Here's how the part is built. I have some questions about the finished solid (model axes, mm). Face numbers are marked on the shaded views. Round coordinates to 2 decimals unless told otherwise and drop trailing zeros. Write each loop counter-clockwise with the first axis right and the second up, starting at its lowest first coordinate (ties: lowest second). Pieces come first, ordered by that corner, then holes. Notation, with made-up numbers: M -12.5,32.5 L 15.5,32.5 A19 cw 15.5,54.5 Z; hole C -10,72.5 d1. An arc over 180 degrees is marked long. Use one line per item in the form item = value. Start each with the question number.
Q1. I want a section at A-A on z = 0. List the corners of the cut face in (x, y) for me.
Q2. I'm going to push flat-ended pins straight in: pin 1 Ø10 at (x, y) = (16.5, 10) entering from +Z; pin 2 Ø6 at (x, y) = (-25, 31) entering from +Z; pin 3 Ø6 at (x, z) = (0, 0) entering from -Y. Where does each tip first touch, or does it pass through?
Q3. I want a section at C-C on x = 16. List the corners of the cut face in (y, z) for me, and give its area (3 significant figures).
Q4. I want a section at D-D on y = 32.5. List the corners of the cut face in (x, z) for me, and give its area (3 significant figures).
Q5. I need wall thicknesses on line 1 along X through (y, z) = (37.25, 0); line 2 along X through (y, z) = (7, 0); line 3 along X through (y, z) = (23, 1). Which ranges of each line are inside material? Lowest first, please. Write a range as from..to.
Q6. We'd pull the mould along Z, two halves only. Please class the marked faces 1, 2, 3 and 4: +Z half, -Z half, draft (parallel to the pull), parting line (faces both ways), or undercut.
Q7. I want a section at B-B on y = 47. List the corners of the cut face in (x, z) for me, and give its area (3 significant figures).
```python
from build123d import *

# Parameters (mm, degrees)
ESQUISSE1_R              = 47.75
BOSS_EXTRU_1_DEPTH       = 50
ESQUISSE2_R              = 26
ENL_V_MAT_EXTRU_1_DEPTH  = 20
ESQUISSE3_R              = 11
ENL_V_MAT_EXTRU_5_DEPTH  = 7.5
ESQUISSE4_R              = 5
ENL_V_MAT_EXTRU_6_DEPTH  = 13.5
ESQUISSE11_R             = 2.75
ENL_V_MAT_EXTRU_11_DEPTH = 85.024549984
ESQUISSE12_R             = 47.75
ESQUISSE12_R_2           = 46.5
ENL_V_MAT_EXTRU_12_DEPTH = 85.024549984


with BuildPart() as part:
    # Esquisse1 → Boss.-Extru.1 (new body)
    with BuildSketch(Plane(origin=(0, 0, 0), x_dir=(1, 0, 0), z_dir=(0, 1, 0))):
        with Locations(Location((0, 0, 0), (0, 0, 270))):
            Circle(ESQUISSE1_R)
    extrude(amount=BOSS_EXTRU_1_DEPTH)

    # Esquisse2 → Enlèv. mat.-Extru.1 (cut)
    with BuildSketch(Plane(origin=(0, 0, 0), x_dir=(-1, 0, 0), z_dir=(0, -1, 0))):
        with Locations(Location((0, 0, 0), (0, 0, 90))):
            Circle(ESQUISSE2_R)
    extrude(amount=-ENL_V_MAT_EXTRU_1_DEPTH, mode=Mode.SUBTRACT)

    # Esquisse3 → Enlèv. mat.-Extru.5 (cut)
    with BuildSketch(Plane(origin=(0, 20, 0), x_dir=(-1, 0, 0), z_dir=(0, -1, 0))):
        with Locations(Location((0, 0, 0), (0, 0, 90))):
            Circle(ESQUISSE3_R)
    extrude(amount=-ENL_V_MAT_EXTRU_5_DEPTH, mode=Mode.SUBTRACT)

    # Esquisse4 → Enlèv. mat.-Extru.6 (cut)
    with BuildSketch(Plane(origin=(0, 27.5, 0), x_dir=(-1, 0, 0), z_dir=(0, -1, 0))):
        with Locations(Location((0, 0, 0), (0, 0, 90))):
            Circle(ESQUISSE4_R)
    extrude(amount=-ENL_V_MAT_EXTRU_6_DEPTH, mode=Mode.SUBTRACT)

    # Esquisse11 → Enlèv. mat.-Extru.11 (cut, through all)
    with BuildSketch(Plane(origin=(0, 50, 0), x_dir=(1, 0, 0), z_dir=(0, 1, 0))):
        with Locations(Location((-16, 0, 0), (0, 0, 270))):
            Circle(ESQUISSE11_R)
        with Locations(Location((0, 16, 0), (0, 0, 270))):
            Circle(ESQUISSE11_R)
        with Locations(Location((16, 0, 0), (0, 0, 270))):
            Circle(ESQUISSE11_R)
        with Locations(Location((0, -16, 0), (0, 0, 270))):
            Circle(ESQUISSE11_R)
    extrude(amount=-ENL_V_MAT_EXTRU_11_DEPTH, mode=Mode.SUBTRACT)

    # Esquisse12 → Enlèv. mat.-Extru.12 (cut, through all)
    with BuildSketch(Plane.XZ):
        Circle(ESQUISSE12_R)
        with Locations(Location((0, 0, 0), (0, 0, 270))):
            Circle(ESQUISSE12_R_2, mode=Mode.SUBTRACT)
    extrude(amount=-ENL_V_MAT_EXTRU_12_DEPTH, mode=Mode.SUBTRACT)


solid = part.part
```
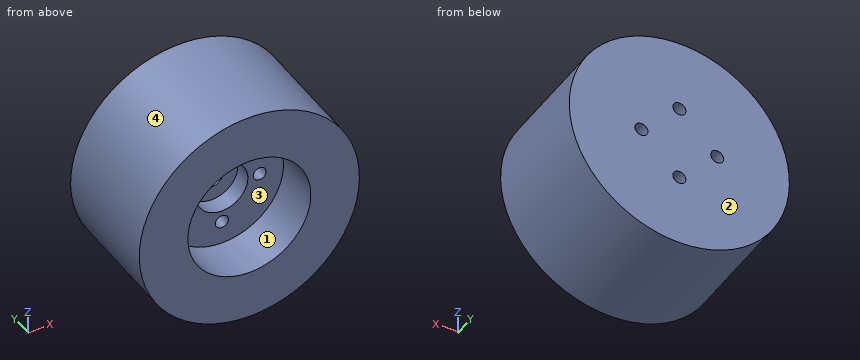
Reported:
q1.outline = M -46.5,0 L -26,0 L -26,20 L -18.75,20 L -18.75,50 L -46.5,50 Z; M -13.25,20 L -11,20 L -11,27.5 L -5,27.5 L -5,41 L 5,41 L 5,27.5 L 11,27.5 L 11,20 L 13.25,20 L 13.25,50 L -13.25,50 Z; M 18.75,20 L 26,20 L 26,0 L 46.5,0 L 46.5,50 L 18.75,50 Z
q2.pin_1 = 45.06
q2.pin_2 = 40.97
q2.pin_3 = 41
q3.outline = M 0,-43.66 L 50,-43.66 L 50,-2.75 L 20,-2.75 L 20,-20.49 L 0,-20.49 Z; M 0,20.49 L 20,20.49 L 20,2.75 L 50,2.75 L 50,43.66 L 0,43.66 Z
q3.area = 3,380 mm^2
q4.outline = C 0,0 d93; hole C -16,0 d5.5; hole C 0,0 d10; hole C 0,-16 d5.5; hole C 0,16 d5.5; hole C 16,0 d5.5
q4.area = 6,620 mm^2
q5.line_1 = -46.5..-18.75, -13.25..-5, 5..13.25, 18.75..46.5
q5.line_2 = -46.5..-26, 26..46.5
q5.line_3 = -46.49..-18.56, -13.44..-10.95, 10.95..13.44, 18.56..46.49
q6.face_1 = undercut
q6.face_2 = draft
q6.face_3 = undercut
q6.face_4 = parting line
q7.outline = C 0,0 d93; hole C -16,0 d5.5; hole C 0,-16 d5.5; hole C 0,16 d5.5; hole C 16,0 d5.5
q7.area = 6,700 mm^2
